from build123d import *

# Parameters (mm, degrees)
EXTRUDE_1_DEPTH = 400


with BuildPart() as part:
    # Эскиз1 → Бобышка-Вытянуть1 (new body)
    with BuildSketch(Plane.XY):
        with BuildLine():
            ThreePointArc((-10.65, 15), (-13.725914498, 13.725914498), (-15, 10.65))
            Line((-15, 10.65), (-15, 4.2))
            Line((-15, 4.2), (-13.6, 4.2))
            Line((-13.6, 4.2), (-13.6, 11))
            ThreePointArc((-13.6, 11), (-13.457683666, 11.620521732), (-13.186420313, 12.196470819))
            Line((-13.186420313, 12.196470819), (-7.487867966, 6.497918472))
            ThreePointArc((-7.487867966, 6.497918472), (-7.42283614, 6.400591467), (-7.4, 6.285786438))
            Line((-7.4, 6.285786438), (-7.4, 0))
            Line((-7.4, 0), (-7.4, -6.285786438))
            ThreePointArc((-7.4, -6.285786438), (-7.42283614, -6.400591467), (-7.487867966, -6.497918472))
            Line((-7.487867966, -6.497918472), (-13.186420313, -12.196470819))
            ThreePointArc((-13.186420313, -12.196470819), (-13.457683666, -11.620521732), (-13.6, -11))
            Line((-13.6, -11), (-13.6, -4.2))
            Line((-13.6, -4.2), (-15, -4.2))
            Line((-15, -4.2), (-15, -10.65))
            ThreePointArc((-15, -10.65), (-13.725914498, -13.725914498), (-10.65, -15))
            Line((-10.65, -15), (-4.2, -15))
            Line((-4.2, -15), (-4.2, -13.6))
            Line((-4.2, -13.6), (-11, -13.6))
            ThreePointArc((-11, -13.6), (-11.620521732, -13.457683666), (-12.196470819, -13.186420313))
            Line((-12.196470819, -13.186420313), (-6.497918472, -7.487867966))
            ThreePointArc((-6.497918472, -7.487867966), (-6.400591467, -7.42283614), (-6.285786438, -7.4))
            Line((-6.285786438, -7.4), (6.285786438, -7.4))
            ThreePointArc((6.285786438, -7.4), (6.400591467, -7.42283614), (6.497918472, -7.487867966))
            Line((6.497918472, -7.487867966), (12.196470819, -13.186420313))
            ThreePointArc((12.196470819, -13.186420313), (11.620521732, -13.457683666), (11, -13.6))
            Line((11, -13.6), (4.2, -13.6))
            Line((4.2, -13.6), (4.2, -15))
            Line((4.2, -15), (10.65, -15))
            ThreePointArc((10.65, -15), (13.725914498, -13.725914498), (15, -10.65))
            Line((15, -10.65), (15, -4.2))
            Line((15, -4.2), (13.6, -4.2))
            Line((13.6, -4.2), (13.6, -11))
            ThreePointArc((13.6, -11), (13.457683666, -11.620521732), (13.186420313, -12.196470819))
            Line((13.186420313, -12.196470819), (7.487867966, -6.497918472))
            ThreePointArc((7.487867966, -6.497918472), (7.42283614, -6.400591467), (7.4, -6.285786438))
            Line((7.4, -6.285786438), (7.4, 0))
            Line((7.4, 0), (7.4, 6.285786438))
            ThreePointArc((7.4, 6.285786438), (7.42283614, 6.400591467), (7.487867966, 6.497918472))
            Line((7.487867966, 6.497918472), (13.186420313, 12.196470819))
            ThreePointArc((13.186420313, 12.196470819), (13.457683666, 11.620521732), (13.6, 11))
            Line((13.6, 11), (13.6, 4.2))
            Line((13.6, 4.2), (15, 4.2))
            Line((15, 4.2), (15, 10.65))
            ThreePointArc((15, 10.65), (13.725914498, 13.725914498), (10.65, 15))
            Line((10.65, 15), (4.2, 15))
            Line((4.2, 15), (4.2, 13.6))
            Line((4.2, 13.6), (11, 13.6))
            ThreePointArc((11, 13.6), (11.620521732, 13.457683666), (12.196470819, 13.186420313))
            Line((12.196470819, 13.186420313), (6.497918472, 7.487867966))
            ThreePointArc((6.497918472, 7.487867966), (6.400591467, 7.42283614), (6.285786438, 7.4))
            Line((6.285786438, 7.4), (0, 7.4))
            Line((0, 7.4), (-6.285786438, 7.4))
            ThreePointArc((-6.285786438, 7.4), (-6.400591467, 7.42283614), (-6.497918472, 7.487867966))
            Line((-6.497918472, 7.487867966), (-12.196470819, 13.186420313))
            ThreePointArc((-12.196470819, 13.186420313), (-11.620521732, 13.457683666), (-11, 13.6))
            Line((-11, 13.6), (-4.2, 13.6))
            Line((-4.2, 13.6), (-4.2, 15))
            Line((-4.2, 15), (-10.65, 15))
        make_face()
        with BuildLine():
            Line((0.01702519, 6.2), (5.9, 6.2))
            ThreePointArc((5.9, 6.2), (6.112132034, 6.112132034), (6.2, 5.9))
            Line((6.2, 5.9), (6.2, -0.01702519))
            Line((6.2, -0.01702519), (6.2, -5.9))
            ThreePointArc((6.2, -5.9), (6.112132034, -6.112132034), (5.9, -6.2))
            Line((5.9, -6.2), (0.01702519, -6.2))
            Line((0.01702519, -6.2), (-0.01702519, -6.2))
            Line((-0.01702519, -6.2), (-5.9, -6.2))
            ThreePointArc((-5.9, -6.2), (-6.112132034, -6.112132034), (-6.2, -5.9))
            Line((-6.2, -5.9), (-6.2, -0.01702519))
            Line((-6.2, -0.01702519), (-6.2, 0))
            Line((-6.2, 0), (-6.2, 5.9))
            ThreePointArc((-6.2, 5.9), (-6.112132034, 6.112132034), (-5.9, 6.2))
            Line((-5.9, 6.2), (0, 6.2))
            Line((0, 6.2), (0.01702519, 6.2))
        make_face(mode=Mode.SUBTRACT)
    extrude(amount=EXTRUDE_1_DEPTH)


solid = part.part
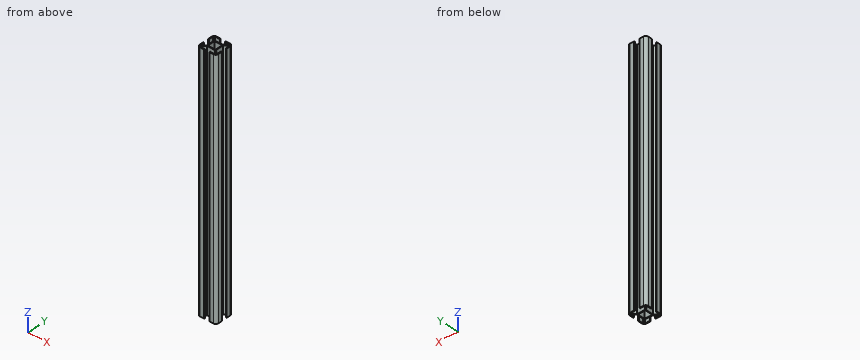
Work out the finished part from the listing and answer in its coordinate system (mm). Round coordinates to 2 decimals unless told otherwise and drop trailing zeros. Write each loop counter-clockwise with the first axis right and the second up, starting at its lowest first coordinate (ties: lowest second). Pieces come first, ordered by that corner, then holes. Notation, with made-up numbers: (28, 24) - (36, 24) arc R14 cw to (36, 28) - close; hole circle Ø10 at (17.25, 63.5). An arc over 180 degrees is marked (long way). Answer in a Markdown table with one row per item. Add a question column.
1. Given pin 1 (13 mm diameter, centred on y = 2.5, z = 119.5, fed in from -X); pin 2 (1.5 mm diameter, centred on y = -1.5, z = 52.5, fed in from +X); pin 3 (1.1 mm diameter, centred on x = 14.5, z = 254.5, fed in from +Y); pin 4 (2 mm diameter, centred on y = 0, z = 167, fed in from -X), each flat-ended and moving along its own axis, determine where each tip first touches the part or whether it passes through.
2. A cutting plane is placed at A-A, the plane x = 0.5. Determine the outline of the cut face in (y, z), and give its area (3 significant figures).
3. Find the intervals of material crossed by line 1 along X through (y, z) = (4.75, 256.5); line 2 along X through (y, z) = (-1.5, 135.5), in increasing order. Write a range as from..to.
Worked out:
| question | item | result |
|---|---|---|
| 1 | pin 1 | x = -15 |
| 1 | pin 2 | x = 7.4 |
| 1 | pin 3 | y = 13.48 |
| 1 | pin 4 | x = -7.4 |
| 2 | outline | (-7.4, 0) - (-6.2, 0) - (-6.2, 400) - (-7.4, 400) - close; (6.2, 0) - (7.4, 0) - (7.4, 400) - (6.2, 400) - close |
| 2 | area | 960 mm^2 |
| 3 | line 1 | -15..-13.6, -7.4..-6.2, 6.2..7.4, 13.6..15 |
| 3 | line 2 | -7.4..-6.2, 6.2..7.4 |
